Check sheet for the modelled part. Datum: model origin and axes. Units: mm. Face numbers are marked on the shaded views. A direction names the side the tool comes from. Round coordinates to 2 decimals unless told otherwise and drop trailing zeros. Order: outer loops, then holes, each group sorted by start corner. A loop starts at its lowest first (then second) coordinate and runs counter-clockwise, first axis right, second up.
(1) Tool access check on the marked faces 1 and 2. Record the directions out of +Z, -Z, +X, -X, +Y, -Y that give a thin tool (end or side, any length) a straight path to the whole face; none if there is none.
(2) Sectioned sample at D-D, the plane y = -19. Enter the section's corners in (x, z), and give its area (3 significant figures).
(3) Thickness scan on probe 1 along Y at (x, z) = (-11.25, 1.3); probe 2 along Y at (x, z) = (-21.25, -0.1); probe 3 along X at (y, z) = (-19, -0.5). Record the ranges inside material, lowest first.
(4) Sectioned sample at A-A, the plane x = -31.25. Enter the section's corners in (y, z), and give its area (3 significant figures).
(5) Mould release check, pull along X, two halves, no side actions. Record for the marked faces 3, 4 and 5: released by +X, released by -X, zero draft, split by the parting line, or undercut.
(6) Sectioned sample at C-C, the plane z = 1.25. Enter the section's corners in (x, y), and give its area (3 significant figures).
(7) Depth check by flat-ended pin: pin 1 (1.8 mm diameter, centred on y = -20.5, z = 0.5, fed in from -X); pin 2 (2 mm diameter, centred on x = 28, z = 1.5, fed in from -Y); pin 3 (3 mm diameter, centred on y = -20.5, z = 1, fed in from +X). Enter the tip coordinate at first touch or a pass-through.
(8) Sectioned sample at B-B, the plane y = 5. Enter the section's corners in (x, z), and give its area (3 significant figures).
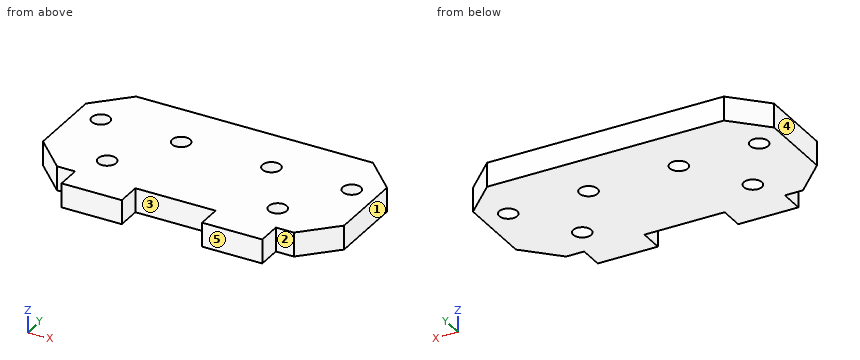
```python
from build123d import *

# Parameters (mm, degrees)
CROQUIS1_W                   = 75
CROQUIS1_H                   = 35
CROQUIS1_R                   = 2.25
SALIENTE_EXTRUIR1_DEPTH      = 3
TALADRO_DE_MARGEN_PARA_M41_D = 4.5
CROQUIS6_W                   = 15
CROQUIS6_H                   = 6
SALIENTE_EXTRUIR2_DEPTH      = 6
CHAFL_N1_SIZE                = 8


with BuildPart() as part:
    # Croquis1 → Saliente-Extruir1 (new, symmetric)
    with BuildSketch(Plane.XY):
        Rectangle(CROQUIS1_W, CROQUIS1_H)
        with Locations((-11.25, 5)):
            Circle(CROQUIS1_R, mode=Mode.SUBTRACT)
    extrude(amount=SALIENTE_EXTRUIR1_DEPTH, both=True)

    # Taladro de margen para M41 (through all)
    with Locations(Plane.XY.offset(3)):
        with Locations((-31.25, 5), (31.25, 5), (11.25, 5), (-21.25, -10), (21.25, -10)):
            Hole(TALADRO_DE_MARGEN_PARA_M41_D / 2)

    # Croquis6 → Saliente-Extruir2 (add, through all)
    with BuildSketch(Plane.XY.offset(3)):
        with Locations((-17.5, -20.5)):
            Rectangle(CROQUIS6_W, CROQUIS6_H)
        with Locations((17.5, -20.5)):
            Rectangle(CROQUIS6_W, CROQUIS6_H)
    extrude(amount=-SALIENTE_EXTRUIR2_DEPTH)

    # Chaflán1
    chafl_n1_edges = [part.edges().sort_by_distance(p)[0] for p in [
        (-37.5, 17.5, 0),
        (37.5, 17.5, 0),
        (37.5, -17.5, 0),
        (-37.5, -17.5, 0),
    ]]
    chamfer(chafl_n1_edges, length=CHAFL_N1_SIZE)


solid = part.part
```
Derived:
1. face 1: +Z, -Z, +X, +Y, -Y
1. face 2: +Z, -Z, +X, -Y
2. outline: (-25, -3) - (-10, -3) - (-10, 3) - (-25, 3) - close; (10, -3) - (25, -3) - (25, 3) - (10, 3) - close
2. area: 180 mm2
3. probe 1: y = -23.5 to 2.75, 7.25 to 17.5
3. probe 2: y = -23.5 to -12.25, -7.75 to 17.5
3. probe 3: x = -25 to -10, 10 to 25
4. outline: (-15.75, -3) - (2.75, -3) - (2.75, 3) - (-15.75, 3) - close; (7.25, -3) - (15.75, -3) - (15.75, 3) - (7.25, 3) - close
4. area: 162 mm2
5. face 3: undercut
5. face 4: released by -X
5. face 5: zero draft
6. outline: (-37.5, -9.5) - (-29.5, -17.5) - (-25, -17.5) - (-25, -23.5) - (-10, -23.5) - (-10, -17.5) - (10, -17.5) - (10, -23.5) - (25, -23.5) - (25, -17.5) - (29.5, -17.5) - (37.5, -9.5) - (37.5, 9.5) - (29.5, 17.5) - (-29.5, 17.5) - (-37.5, 9.5) - close; hole circle Ø4.5 at (-31.25, 5); hole circle Ø4.5 at (-21.25, -10); hole circle Ø4.5 at (-11.25, 5); hole circle Ø4.5 at (11.25, 5); hole circle Ø4.5 at (21.25, -10); hole circle Ø4.5 at (31.25, 5)
6. area: 2,580 mm2
7. pin 1: stops at x = -25
7. pin 2: stops at y = -17.5
7. pin 3: stops at x = 25
8. outline: (-37.5, -3) - (-33.5, -3) - (-33.5, 3) - (-37.5, 3) - close; (-29, -3) - (-13.5, -3) - (-13.5, 3) - (-29, 3) - close; (-9, -3) - (9, -3) - (9, 3) - (-9, 3) - close; (13.5, -3) - (29, -3) - (29, 3) - (13.5, 3) - close; (33.5, -3) - (37.5, -3) - (37.5, 3) - (33.5, 3) - close
8. area: 342 mm2
